Source: CAD feature listing. Evaluate the final solid. Frame: model axes, mm. Face numbers are marked on the shaded views. A direction names the side the tool comes from. Give positions to 0.01 mm unless a question says otherwise; leave off trailing zeros. Order: outer loops, then holes, each group sorted by start corner. A loop starts at its lowest first (then second) coordinate and runs counter-clockwise, first axis right, second up. Notation, with made-up numbers: (-32.75, 81) - (9.25, 81) arc R24 cw to (9.25, 111) - close; hole circle Ø2 at (-14.75, -33). An arc over 180 degrees is marked (long way). Write each question's results on one line, items separated by ' | '. Start each with the question number.
Item 1: Set-up query: the marked faces 4, 5 and 6. Return all of +Z, -Z, +X, -X, +Y, -Y with unobstructed straight access to the full face (end or side cutting, diameter ignored); none if empty.
Item 2: Section A-A on z = 86.6. Output: boundary loops of the cut face in (x, y).
Item 3: Section B-B on x = -59.5. Output: boundary loops of the cut face in (y, z) (3 decimals).
Item 4: Line query: line 1 along Z through (x, y) = (-53.75, -84.2); line 2 along Y through (x, z) = (-59.5, 85.95); line 3 along X through (y, z) = (-74.6, 86.75). Output: solid intervals per line, ascending.
Item 5: Contact query for flat-ended pins moving along their axis: pin 1 Ø3 at (x, y) = (-57, -74.5) entering from +Z; pin 2 Ø2 at (x, y) = (-59.5, -74.6) entering from +Z; pin 3 Ø10 at (x, y) = (-61.5, -80) entering from +Z (3 decimals). Output: stop coordinate, or through.
Item 6: Mould query, pull axis Y, two halves, no side actions, for the marked faces 1, 2 and 3. Classes: released by +Y, released by -Y, zero draft, split by the parting line, or undercut.
```python
from build123d import *

# Parameters (mm, degrees)
PAD011_DEPTH    = 5.3
SKETCH027_W     = 31.062653
SKETCH027_H     = 8.215561
POCKET012_DEPTH = 0.305
FILLET005_R     = 2.45
FILLET006_R     = 1
SKETCH028_R     = 9
POCKET013_DEPTH = 1
SKETCH029_R     = 1.65
POCKET014_DEPTH = 5
SKETCH030_R     = 1.5
POCKET015_DEPTH = 31
CHAMFER001_SIZE = 1


with BuildPart() as part:
    # Sketch026 → Pad011 (new body)
    with BuildSketch(Plane.XY):
        with BuildLine():
            ThreePointArc((15, 0), (0, 15), (-15, 0))
            Line((-15, 0), (-15, -12))
            Line((-15, -12), (15, -12))
            Line((15, 0), (15, -12))
        make_face()
    extrude(amount=PAD011_DEPTH)

    # Sketch027 (on Face6 of Pad011) → Pocket012 (cut)
    with BuildSketch(Plane.XY.offset(5.3)):
        with Locations((0.051316, -9.153541)):
            Rectangle(SKETCH027_W, SKETCH027_H)
    extrude(amount=-POCKET012_DEPTH, mode=Mode.SUBTRACT)

    # Fillet005
    fillet005_edges = [part.edges().sort_by_distance(p)[0] for p in [
        (0, -12, 4.995),
    ]]
    fillet(fillet005_edges, radius=FILLET005_R)

    # Fillet006
    fillet006_edges = [part.edges().sort_by_distance(p)[0] for p in [
        (0, 15, 5.3),
    ]]
    fillet(fillet006_edges, radius=FILLET006_R)

    # Sketch028 (on Face12 of Fillet006) → Pocket013 (cut)
    with BuildSketch(Plane.XY.offset(5.3)):
        Circle(SKETCH028_R)
    extrude(amount=-POCKET013_DEPTH, mode=Mode.SUBTRACT)

    # Sketch029 (on Face15 of Pocket013) → Pocket014 (cut)
    with BuildSketch(Plane.XY.offset(4.3)):
        Circle(SKETCH029_R)
    extrude(amount=-POCKET014_DEPTH, mode=Mode.SUBTRACT)

    # Sketch030 (on Face1 of Pocket014) → Pocket015 (cut)
    with BuildSketch(Plane.YZ.offset(15)):
        with Locations((-9.6, 2.5)):
            Circle(SKETCH030_R)
    extrude(amount=-POCKET015_DEPTH, mode=Mode.SUBTRACT)

    # Chamfer001
    chamfer001_edges = [part.edges().sort_by_distance(p)[0] for p in [
        (-1.65, 0, 4.3),
    ]]
    chamfer(chamfer001_edges, length=CHAMFER001_SIZE)


with BuildPart() as part_1:
    # Body007 placement: moved
    add(part.part.moved(Location((-59.5, -74.6, 85))))


solid = part_1.part
```
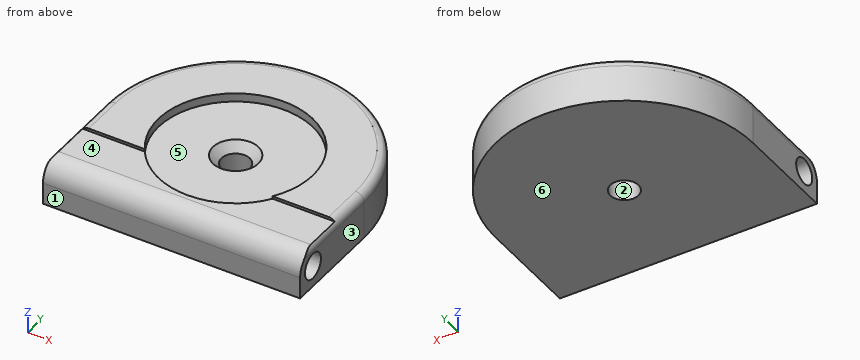
Evaluation:
1) face 4: +Z, +X, -X, -Y | face 5: +Z | face 6: -Z, +X, -X, +Y, -Y
2) outline: (-74.5, -86.6) - (-44.5, -86.6) - (-44.5, -85.4) - (-74.5, -85.4) - close; (-74.5, -83) - (-44.5, -83) - (-44.5, -74.6) arc R15 ccw to (-74.5, -74.6) - close; hole circle Ø3.3 at (-59.5, -74.6)
3) outline: (-86.6, 85) - (-76.25, 85) - (-76.25, 88.3) - (-77.25, 89.3) - (-83.6, 89.3) - (-83.6, 89.995) - (-84.15, 89.995) arc R2.45 ccw to (-86.6, 87.545) - close; (-72.95, 85) - (-59.6, 85) - (-59.6, 89.3) arc R1 ccw to (-60.6, 90.3) - (-65.6, 90.3) - (-65.6, 89.3) - (-71.95, 89.3) - (-72.95, 88.3) - close; hole circle Ø3 at (-84.2, 87.5)
4) line 1: z = 85 to 86, 89 to 89.99 | line 2: y = -86.6 to -76.25, -72.95 to -59.6 | line 3: x = -74.5 to -61.15, -57.85 to -44.5
5) pin 1: stops at z = 89.3 | pin 2: passes through | pin 3: stops at z = 89.995
6) face 1: released by -Y | face 2: undercut | face 3: zero draft
